```python
from build123d import *

# Parameters (mm, degrees)
SKETCH1_R           = 3.81
BOSS_EXTRUDE1_DEPTH = 1.27


with BuildPart() as part:
    # Sketch1 → Boss-Extrude1 (new, symmetric)
    with BuildSketch(Plane.YZ):
        with BuildLine():
            Line((141.141238808, -800.451741648), (141.93592589, -805.469198419))
            Line((141.93592589, -805.469198419), (129.136650891, -815.336725161))
            ThreePointArc((129.136650891, -815.336725161), (0, -825.5), (-129.136650891, -815.336725161))
            Line((-129.136650891, -815.336725161), (-141.93592589, -805.469198419))
            Line((-141.93592589, -805.469198419), (-141.141238808, -800.451741648))
            ThreePointArc((-141.141238808, -800.451741648), (0, -812.8), (141.141238808, -800.451741648))
        make_face()
        with Locations(Location((0, -819.15, 0), (0, 0, 270))):
            Circle(SKETCH1_R, mode=Mode.SUBTRACT)
    extrude(amount=BOSS_EXTRUDE1_DEPTH, both=True)


solid = part.part
```
Work out the finished part from the listing and answer in its coordinate system (mm). Round coordinates to 2 decimals unless told otherwise and drop trailing zeros. Order: outer loops, then holes, each group sorted by start corner. A loop starts at its lowest first (then second) coordinate and runs counter-clockwise, first axis right, second up.
Q1. A cutting plane is placed at B-B, the plane x = 0.4. Determine the outline of the cut face in (y, z).
Solution:
outline: (-141.94, -805.47) - (-129.14, -815.34) arc R825.5 ccw to (129.14, -815.34) - (141.94, -805.47) - (141.14, -800.45) arc R812.8 cw to (-141.14, -800.45) - close; hole circle Ø7.62 at (0, -819.15)
Q2. A cutting plane is placed at D-D, the plane y = -87. Determine the outline of the cut face in (x, z).
Solution:
outline: (-1.27, -820.9) - (1.27, -820.9) - (1.27, -808.13) - (-1.27, -808.13) - close
Q3. A cutting plane is placed at A-A, the plane y = 0. Determine the outline of the cut face in (x, z).
Solution:
outline: (-1.27, -825.5) - (1.27, -825.5) - (1.27, -822.96) - (-1.27, -822.96) - close; (-1.27, -815.34) - (1.27, -815.34) - (1.27, -812.8) - (-1.27, -812.8) - close
Q4. The mould has two halves that part along Z. Classify faces 1 (the flat face through (-1.27, 2, -815.6)), 2 (the cylindrical face through (-0.018, 0.168, -815.344)), 3 (the cylindrical face through (0, 1.8, -825.5)): pulls with the +Z half, pulls with the -Z half, needs draft (parallel to the pull), parting line crosses it, or undercut.
Solution:
face 1: needs draft
face 2: undercut
face 3: pulls with the -Z half
Q5. Find the intervals of material crossed by line 1 along Z through (x, y) = (-0.2, 86); line 2 along Z through (x, y) = (1.15, 99); line 3 along Y through (x, z) = (-0.85, -814.5), in increasing order.
Solution:
line 1: z = -821.01 to -808.24
line 2: z = -819.54 to -806.75
line 3: y = -130.22 to 130.22
